Read the model definition and answer for the solid it produces. Units are mm, in the model's axes. A direction names the side the tool comes from. Round coordinates to 2 decimals unless told otherwise and drop trailing zeros. Loops run counter-clockwise (first coordinate to the right, second up) from the corner with the lowest first, then second, coordinate; pieces in that order, holes last. Notation, with made-up numbers: (85, 49) - (98, 49) arc R26 cw to (98, 66) - close; hole circle Ø8 at (55, 80.5). An arc over 180 degrees is marked (long way). Use CSV: the item, a comma, the result in double quotes. Start each with the question number.
1. Determine the mould class of faces 1 (the flat face through (30, 0, -195)), 2 (the cylindrical face through (105.886, 2.465, -239.521)), 3 (the flat face through (87, 5, -321.979)) for opening direction Z: +Z half, -Z half, draft (parallel to the pull), parting line (faces both ways), or undercut.
2. A tool of negligible diameter and unlimited length cuts with its end or side. For faces 4 (the flat face through (159, 6, -296.979)), 5 (the cylindrical face through (144.443, 2.465, -21.721)), from which of +Z, -Z, +X, -X, +Y, -Y can it reach the whole face along a straight path? Write none if from no direction.
3. Find section A-A (z = -215). State how many separate pieces and enclosed holes the cut face has, and give its area (3 significant figures).
4. Find section B-B (y = 16). Give the vertices of the cut face in (x, z) (3 decimals).
5. Given pin 1 Ø17.5 at (x, z) = (153.61, -15.88) entering from -Y; pin 2 Ø3 at (x, y) = (57.5, 11.5) entering from -Z; pin 3 Ø10 at (x, z) = (69.5, -180.5) entering from +Y; pin 4 Ø14 at (x, z) = (67, -305.5) entering from +Y, each flat-ended and moving along its own axis, determine where each tip first touches the part or whether it passes through.
6. Consider line 1 along Z through (x, y) = (49, 18.75); line 2 along Z through (x, y) = (100.5, 8); line 3 along Y through (x, z) = (31.5, -160.5). Determine where each line is inside the solid, lowest interval first.
from build123d import *

# Parameters (mm, degrees)
SKETCH2_W            = 171.7
SKETCH2_H            = 290.628679219
BOSS_EXTRUDE6_DEPTH  = 5
SKETCH1_R            = 10.875
CUT_EXTRUDE1_DEPTH   = 7
SKETCH5_R            = 3.3
CUT_EXTRUDE3_DEPTH   = 5
SKETCH12_W           = 171.7
SKETCH12_H           = 20
BOSS_EXTRUDE9_DEPTH  = 6.35
SKETCH13_W           = 153.01
SKETCH13_H           = 11
CUT_EXTRUDE7_DEPTH   = 3.18
SKETCH14_W           = 129.7
SKETCH14_H           = 9
BOSS_EXTRUDE10_DEPTH = 25
FILLET1_R            = 7


with BuildPart() as part:
    # Sketch2 → Boss-Extrude6 (new body)
    with BuildSketch(Plane(origin=(0, 0, 0), x_dir=(1, 0, 0), z_dir=(0, 1, 0))):
        with Locations((85.85, 145.314339609)):
            Rectangle(SKETCH2_W, SKETCH2_H)
    extrude(amount=BOSS_EXTRUDE6_DEPTH)

    # Sketch1 → Cut-Extrude1 (cut)
    with BuildSketch(Plane(origin=(0, 0, 0), x_dir=(1, 0, 0), z_dir=(0, 1, 0))):
        with Locations(Location((130.663177129, 15.875, 0), (0, 0, 90))):
            Circle(SKETCH1_R)
        with Locations(Location((153.613177129, 15.875, 0), (0, 0, 90))):
            Circle(SKETCH1_R)
        with Locations(Location((142.138177129, 35.750283017, 0), (0, 0, 90))):
            Circle(SKETCH1_R)
        with Locations(Location((119.188177129, 35.750283017, 0), (0, 0, 90))):
            Circle(SKETCH1_R)
        with Locations(Location((96.238177129, 35.750283017, 0), (0, 0, 90))):
            Circle(SKETCH1_R)
        with Locations(Location((107.713177129, 55.625566034, 0), (0, 0, 90))):
            Circle(SKETCH1_R)
        with Locations(Location((130.663177129, 55.625566034, 0), (0, 0, 90))):
            Circle(SKETCH1_R)
        with Locations(Location((153.613177129, 55.625566034, 0), (0, 0, 90))):
            Circle(SKETCH1_R)
        with Locations(Location((142.138177129, 75.500849051, 0), (0, 0, 90))):
            Circle(SKETCH1_R)
        with Locations(Location((119.188177129, 75.500849051, 0), (0, 0, 90))):
            Circle(SKETCH1_R)
        with Locations(Location((96.238177129, 75.500849051, 0), (0, 0, 90))):
            Circle(SKETCH1_R)
        with Locations(Location((107.713177129, 95.376132067, 0), (0, 0, 90))):
            Circle(SKETCH1_R)
        with Locations(Location((130.663177129, 95.376132067, 0), (0, 0, 90))):
            Circle(SKETCH1_R)
        with Locations(Location((153.613177129, 95.376132067, 0), (0, 0, 90))):
            Circle(SKETCH1_R)
        with Locations(Location((142.138177129, 115.251415084, 0), (0, 0, 90))):
            Circle(SKETCH1_R)
        with Locations(Location((119.188177129, 115.251415084, 0), (0, 0, 90))):
            Circle(SKETCH1_R)
        with Locations(Location((96.238177129, 115.251415084, 0), (0, 0, 90))):
            Circle(SKETCH1_R)
        with Locations(Location((107.713177129, 135.126698101, 0), (0, 0, 90))):
            Circle(SKETCH1_R)
        with Locations(Location((130.663177129, 135.126698101, 0), (0, 0, 90))):
            Circle(SKETCH1_R)
        with Locations(Location((153.613177129, 135.126698101, 0), (0, 0, 90))):
            Circle(SKETCH1_R)
        with Locations(Location((142.138177129, 155.001981118, 0), (0, 0, 90))):
            Circle(SKETCH1_R)
        with Locations(Location((119.188177129, 155.001981118, 0), (0, 0, 90))):
            Circle(SKETCH1_R)
        with Locations(Location((96.238177129, 155.001981118, 0), (0, 0, 90))):
            Circle(SKETCH1_R)
        with Locations(Location((107.713177129, 174.877264135, 0), (0, 0, 90))):
            Circle(SKETCH1_R)
        with Locations(Location((96.238177129, 194.752547152, 0), (0, 0, 90))):
            Circle(SKETCH1_R)
        with Locations(Location((107.713177129, 214.627830169, 0), (0, 0, 90))):
            Circle(SKETCH1_R)
        with Locations(Location((96.238177129, 234.503113185, 0), (0, 0, 90))):
            Circle(SKETCH1_R)
        with Locations(Location((107.713177129, 254.378396202, 0), (0, 0, 90))):
            Circle(SKETCH1_R)
        with Locations(Location((96.238177129, 274.253679219, 0), (0, 0, 90))):
            Circle(SKETCH1_R)
        with Locations(Location((119.188177129, 274.253679219, 0), (0, 0, 90))):
            Circle(SKETCH1_R)
        with Locations(Location((142.138177129, 274.253679219, 0), (0, 0, 90))):
            Circle(SKETCH1_R)
        with Locations(Location((153.613177129, 254.378396202, 0), (0, 0, 90))):
            Circle(SKETCH1_R)
        with Locations(Location((130.663177129, 254.378396202, 0), (0, 0, 90))):
            Circle(SKETCH1_R)
        with Locations(Location((119.188177129, 234.503113185, 0), (0, 0, 90))):
            Circle(SKETCH1_R)
        with Locations(Location((142.138177129, 234.503113185, 0), (0, 0, 90))):
            Circle(SKETCH1_R)
        with Locations(Location((130.663177129, 214.627830169, 0), (0, 0, 90))):
            Circle(SKETCH1_R)
        with Locations(Location((153.613177129, 214.627830169, 0), (0, 0, 90))):
            Circle(SKETCH1_R)
        with Locations(Location((142.138177129, 194.752547152, 0), (0, 0, 90))):
            Circle(SKETCH1_R)
        with Locations(Location((153.613177129, 174.877264135, 0), (0, 0, 90))):
            Circle(SKETCH1_R)
        with Locations(Location((130.663177129, 174.877264135, 0), (0, 0, 90))):
            Circle(SKETCH1_R)
        with Locations(Location((119.188177129, 194.752547152, 0), (0, 0, 90))):
            Circle(SKETCH1_R)
        with Locations(Location((63.989741568, 274.253679219, 0), (0, 0, 90))):
            Circle(SKETCH1_R)
        with Locations(Location((41.039741568, 274.253679219, 0), (0, 0, 90))):
            Circle(SKETCH1_R)
        with Locations(Location((18.089741568, 274.253679219, 0), (0, 0, 90))):
            Circle(SKETCH1_R)
        with Locations(Location((29.564741568, 254.378396202, 0), (0, 0, 90))):
            Circle(SKETCH1_R)
        with Locations(Location((52.514741568, 254.378396202, 0), (0, 0, 90))):
            Circle(SKETCH1_R)
        with Locations(Location((75.464741568, 254.378396202, 0), (0, 0, 90))):
            Circle(SKETCH1_R)
        with Locations(Location((63.989741568, 234.503113185, 0), (0, 0, 90))):
            Circle(SKETCH1_R)
        with Locations(Location((41.039741568, 234.503113185, 0), (0, 0, 90))):
            Circle(SKETCH1_R)
        with Locations(Location((29.564741568, 214.627830169, 0), (0, 0, 90))):
            Circle(SKETCH1_R)
        with Locations(Location((18.089741568, 234.503113185, 0), (0, 0, 90))):
            Circle(SKETCH1_R)
        with Locations(Location((52.514741568, 214.627830169, 0), (0, 0, 90))):
            Circle(SKETCH1_R)
        with Locations(Location((75.464741568, 214.627830169, 0), (0, 0, 90))):
            Circle(SKETCH1_R)
        with Locations(Location((63.989741568, 194.752547152, 0), (0, 0, 90))):
            Circle(SKETCH1_R)
        with Locations(Location((41.039741568, 194.752547152, 0), (0, 0, 90))):
            Circle(SKETCH1_R)
        with Locations(Location((18.089741568, 194.752547152, 0), (0, 0, 90))):
            Circle(SKETCH1_R)
        with Locations(Location((75.464741568, 174.877264135, 0), (0, 0, 90))):
            Circle(SKETCH1_R)
        with Locations(Location((63.989741568, 155.001981118, 0), (0, 0, 90))):
            Circle(SKETCH1_R)
        with Locations(Location((52.514741568, 174.877264135, 0), (0, 0, 90))):
            Circle(SKETCH1_R)
        with Locations(Location((29.564741568, 174.877264135, 0), (0, 0, 90))):
            Circle(SKETCH1_R)
        with Locations(Location((41.039741568, 155.001981118, 0), (0, 0, 90))):
            Circle(SKETCH1_R)
        with Locations(Location((75.464741568, 135.126698101, 0), (0, 0, 90))):
            Circle(SKETCH1_R)
        with Locations(Location((52.514741568, 135.126698101, 0), (0, 0, 90))):
            Circle(SKETCH1_R)
        with Locations(Location((29.564741568, 135.126698101, 0), (0, 0, 90))):
            Circle(SKETCH1_R)
        with Locations(Location((18.089741568, 155.001981118, 0), (0, 0, 90))):
            Circle(SKETCH1_R)
        with Locations(Location((18.089741568, 115.251415084, 0), (0, 0, 90))):
            Circle(SKETCH1_R)
        with Locations(Location((41.039741568, 115.251415084, 0), (0, 0, 90))):
            Circle(SKETCH1_R)
        with Locations(Location((63.989741568, 115.251415084, 0), (0, 0, 90))):
            Circle(SKETCH1_R)
        with Locations(Location((75.464741568, 95.376132067, 0), (0, 0, 90))):
            Circle(SKETCH1_R)
        with Locations(Location((52.514741568, 95.376132067, 0), (0, 0, 90))):
            Circle(SKETCH1_R)
        with Locations(Location((29.564741568, 95.376132067, 0), (0, 0, 90))):
            Circle(SKETCH1_R)
        with Locations(Location((41.039741568, 75.500849051, 0), (0, 0, 90))):
            Circle(SKETCH1_R)
        with Locations(Location((18.089741568, 75.500849051, 0), (0, 0, 90))):
            Circle(SKETCH1_R)
        with Locations(Location((63.989741568, 75.500849051, 0), (0, 0, 90))):
            Circle(SKETCH1_R)
        with Locations(Location((75.464741568, 55.625566034, 0), (0, 0, 90))):
            Circle(SKETCH1_R)
        with Locations(Location((52.514741568, 55.625566034, 0), (0, 0, 90))):
            Circle(SKETCH1_R)
        with Locations(Location((29.564741568, 55.625566034, 0), (0, 0, 90))):
            Circle(SKETCH1_R)
        with Locations(Location((18.089741568, 35.750283017, 0), (0, 0, 90))):
            Circle(SKETCH1_R)
        with Locations(Location((41.039741568, 35.750283017, 0), (0, 0, 90))):
            Circle(SKETCH1_R)
        with Locations(Location((63.989741568, 35.750283017, 0), (0, 0, 90))):
            Circle(SKETCH1_R)
        with Locations(Location((75.464741568, 15.875, 0), (0, 0, 90))):
            Circle(SKETCH1_R)
        with Locations(Location((52.514741568, 15.875, 0), (0, 0, 90))):
            Circle(SKETCH1_R)
        with Locations(Location((29.564741568, 15.875, 0), (0, 0, 90))):
            Circle(SKETCH1_R)
        with Locations(Location((107.713177129, 15.875, 0), (0, 0, 90))):
            Circle(SKETCH1_R)
    extrude(amount=CUT_EXTRUDE1_DEPTH, mode=Mode.SUBTRACT)

    # Sketch5 → Cut-Extrude3 (cut)
    with BuildSketch(Plane(origin=(0, 5, 0), x_dir=(1, 0, 0), z_dir=(0, 1, 0))):
        with Locations(Location((9.344870784, 254.378396202, 0), (0, 0, 270))):
            Circle(SKETCH5_R)
        with Locations(Location((162.356588564, 35.750283017, 0), (0, 0, 270))):
            Circle(SKETCH5_R)
        with Locations(Location((162.356588564, 75.500849051, 0), (0, 0, 270))):
            Circle(SKETCH5_R)
        with Locations(Location((162.356588564, 115.251415084, 0), (0, 0, 270))):
            Circle(SKETCH5_R)
        with Locations(Location((162.356588564, 155.001981118, 0), (0, 0, 270))):
            Circle(SKETCH5_R)
        with Locations(Location((162.356588564, 194.752547152, 0), (0, 0, 270))):
            Circle(SKETCH5_R)
        with Locations(Location((162.356588564, 234.503113185, 0), (0, 0, 270))):
            Circle(SKETCH5_R)
        with Locations(Location((162.356588564, 274.253679219, 0), (0, 0, 270))):
            Circle(SKETCH5_R)
        with Locations(Location((9.344870784, 214.627830169, 0), (0, 0, 270))):
            Circle(SKETCH5_R)
        with Locations(Location((9.344870784, 174.877264135, 0), (0, 0, 270))):
            Circle(SKETCH5_R)
        with Locations(Location((9.344870784, 135.126698101, 0), (0, 0, 270))):
            Circle(SKETCH5_R)
        with Locations(Location((9.344870784, 95.376132067, 0), (0, 0, 270))):
            Circle(SKETCH5_R)
        with Locations(Location((9.344870784, 55.625566034, 0), (0, 0, 270))):
            Circle(SKETCH5_R)
        with Locations(Location((9.344870784, 15.875, 0), (0, 0, 270))):
            Circle(SKETCH5_R)
    extrude(amount=-CUT_EXTRUDE3_DEPTH, mode=Mode.SUBTRACT)

    # Sketch12 → Boss-Extrude9 (add)
    with BuildSketch(Plane(origin=(0, 0, -290.628679219), x_dir=(-1, 0, 0), z_dir=(0, 0, -1))):
        with Locations((-85.85, 10)):
            Rectangle(SKETCH12_W, SKETCH12_H)
    extrude(amount=BOSS_EXTRUDE9_DEPTH)

    # Sketch13 → Cut-Extrude7 (cut)
    with BuildSketch(Plane(origin=(0, 0, -296.978679219), x_dir=(-1, 0, 0), z_dir=(0, 0, -1))):
        with Locations((-85.85, 14.5)):
            Rectangle(SKETCH13_W, SKETCH13_H)
    extrude(amount=-CUT_EXTRUDE7_DEPTH, mode=Mode.SUBTRACT)

    # Sketch14 → Boss-Extrude10 (add)
    with BuildSketch(Plane(origin=(0, 0, -296.978679219), x_dir=(-1, 0, 0), z_dir=(0, 0, -1))):
        with Locations((-85.85, 4.5)):
            Rectangle(SKETCH14_W, SKETCH14_H)
    extrude(amount=BOSS_EXTRUDE10_DEPTH)

    # Fillet1
    fillet1_edges = [part.edges().sort_by_distance(p)[0] for p in [
        (171.7, 10, -296.978679219),
        (0, 10, -296.978679219),
        (171.7, 2.5, 0),
        (0, 2.5, 0),
    ]]
    fillet(fillet1_edges, radius=FILLET1_R)


solid = part.part
Filled sheet:
1,face 1,"draft"
1,face 2,"undercut"
1,face 3,"-Z half"
2,face 4,"-Z, +X, +Y, -Y"
2,face 5,"+Y, -Y"
3,separate pieces,"8"
3,enclosed holes,"0"
3,area,"174 mm²"
4,outline,"(0.03, -290.629) arc R7 ccw to (7, -296.979) - (9.345, -296.979) - (9.345, -293.799) - (162.355, -293.799) - (162.355, -296.979) - (164.7, -296.979) arc R7 ccw to (171.67, -290.629) - close"
5,pin 1,"passes through"
5,pin 2,"stops at z = -293.8"
5,pin 3,"stops at y = 5"
5,pin 4,"stops at y = 9"
6,line 1,"z = -293.8 to -290.63"
6,line 2,"z = -321.98 to -290.63"
6,line 3,"y = 0 to 5"
